The model under review builds one solid part; all positions refer to its coordinate system, in mm. Face numbers are marked on the shaded views. A direction names the side the tool comes from. Give positions to 0.01 mm unless a question says otherwise; leave off trailing zeros. Write each loop counter-clockwise with the first axis right and the second up, starting at its lowest first coordinate (ties: lowest second). Pieces come first, ordered by that corner, then holes. Notation, with made-up numbers: (2, 56.25) -> (28, 56.25) arc R22 ccw to (28, 70.25) -> close; hole circle Ø11 at (-8, 53). An arc over 180 degrees is marked (long way). Use CSV: the item, a comma, the result in double quotes.
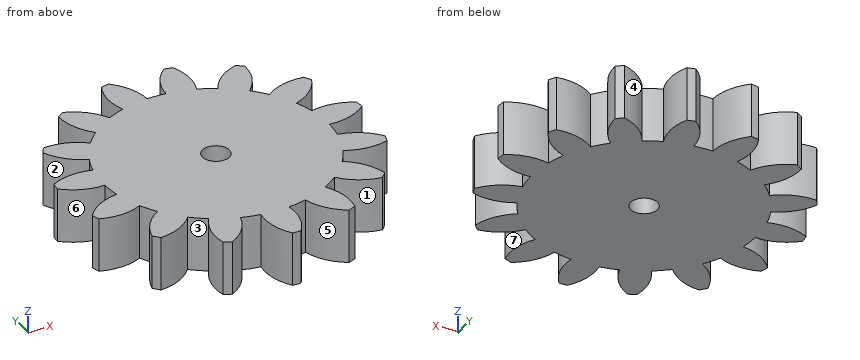
```python
from build123d import *

# Parameters (mm, degrees)
DODANIE_WYCI_GNI_CIE1_DEPTH = 12
OTW_R_6_0_6_1_D             = 6


with BuildPart() as part:
    # Szkic1 → Dodanie-wyciągnięcie1 (new body)
    with BuildSketch(Plane.XY):
        with BuildLine():
            ThreePointArc((-33.898094839, 2.630430818), (-29.769421597, 0.139315972), (-24.993476702, -0.525474417))
            ThreePointArc((-24.993476702, -0.525474417), (-24.862052862, -2.613107053), (-24.556561544, -4.68244446))
            ThreePointArc((-24.556561544, -4.68244446), (-29.089922891, -6.325682363), (-32.610442817, -9.620759807))
            ThreePointArc((-32.610442817, -9.620759807), (-32.335921554, -10.506577809), (-32.037343164, -11.384579176))
            ThreePointArc((-32.037343164, -11.384579176), (-27.252384788, -11.981043133), (-22.618947411, -10.645807579))
            ThreePointArc((-22.618947411, -10.645807579), (-21.649769069, -12.4995), (-20.529013513, -14.265679275))
            ThreePointArc((-20.529013513, -14.265679275), (-24.002080111, -17.610735974), (-25.87800636, -22.052863461))
            ThreePointArc((-25.87800636, -22.052863461), (-25.266924066, -22.750440616), (-24.637043805, -23.431092005))
            ThreePointArc((-24.637043805, -23.431092005), (-20.023163068, -22.029771036), (-16.333396627, -18.925383897))
            ThreePointArc((-16.333396627, -18.925383897), (-14.694043522, -20.224615842), (-12.951812545, -21.382248544))
            ThreePointArc((-12.951812545, -21.382248544), (-14.764059627, -25.850733346), (-14.671027508, -30.671826679))
            ThreePointArc((-14.671027508, -30.671826679), (-13.829045865, -31.06054556), (-12.976775752, -31.426156161))
            ThreePointArc((-12.976775752, -31.426156161), (-9.33175455, -28.269351393), (-7.223653181, -23.932589407))
            ThreePointArc((-7.223653181, -23.932589407), (-5.197584359, -24.452711871), (-3.135125524, -24.801632788))
            ThreePointArc((-3.135125524, -24.801632788), (-2.973199107, -29.620904076), (-0.927294719, -33.98735242))
            ThreePointArc((-0.927294719, -33.98735242), (0, -34), (0.927294719, -33.98735242))
            ThreePointArc((0.927294719, -33.98735242), (2.973199107, -29.620904076), (3.135125524, -24.801632788))
            ThreePointArc((3.135125524, -24.801632788), (5.197584359, -24.452711871), (7.223653181, -23.932589407))
            ThreePointArc((7.223653181, -23.932589407), (9.33175455, -28.269351393), (12.976775752, -31.426156161))
            ThreePointArc((12.976775752, -31.426156161), (13.829045865, -31.06054556), (14.671027508, -30.671826679))
            ThreePointArc((14.671027508, -30.671826679), (14.764059627, -25.850733346), (12.951812545, -21.382248544))
            ThreePointArc((12.951812545, -21.382248544), (14.694043522, -20.224615842), (16.333396627, -18.925383897))
            ThreePointArc((16.333396627, -18.925383897), (20.023163068, -22.029771036), (24.637043805, -23.431092005))
            ThreePointArc((24.637043805, -23.431092005), (25.266924066, -22.750440616), (25.87800636, -22.052863461))
            ThreePointArc((25.87800636, -22.052863461), (24.002080111, -17.610735974), (20.529013513, -14.265679275))
            ThreePointArc((20.529013513, -14.265679275), (21.649769069, -12.4995), (22.618947411, -10.645807579))
            ThreePointArc((22.618947411, -10.645807579), (27.252384788, -11.981043133), (32.037343164, -11.384579176))
            ThreePointArc((32.037343164, -11.384579176), (32.335921554, -10.506577809), (32.610442817, -9.620759807))
            ThreePointArc((32.610442817, -9.620759807), (29.089922891, -6.325682363), (24.556561544, -4.68244446))
            ThreePointArc((24.556561544, -4.68244446), (24.862052862, -2.613107053), (24.993476702, -0.525474417))
            ThreePointArc((24.993476702, -0.525474417), (29.769421597, 0.139315972), (33.898094839, 2.630430818))
            ThreePointArc((33.898094839, 2.630430818), (33.813744443, 3.553967751), (33.704237455, 4.47486062))
            ThreePointArc((33.704237455, 4.47486062), (29.14785373, 6.053139195), (24.338056995, 5.71042754))
            ThreePointArc((24.338056995, 5.71042754), (23.775461851, 7.725115842), (23.046406812, 9.685718046))
            ThreePointArc((23.046406812, 9.685718046), (27.139054966, 12.235586081), (29.897557962, 16.190615427))
            ThreePointArc((29.897557962, 16.190615427), (29.444863729, 17), (28.970263244, 17.796736993))
            ThreePointArc((28.970263244, 17.796736993), (24.165855859, 17.385317995), (19.911281288, 15.115914742))
            ThreePointArc((19.911281288, 15.115914742), (18.577877492, 16.727596028), (17.114403814, 18.222161866))
            ThreePointArc((17.114403814, 18.222161866), (19.81609918, 22.216212199), (20.727461703, 26.951295541))
            ThreePointArc((20.727461703, 26.951295541), (19.984698578, 27.506577809), (19.227067331, 28.041395862))
            ThreePointArc((19.227067331, 28.041395862), (15.00536197, 25.711417373), (12.041664157, 21.907722961))
            ThreePointArc((12.041664157, 21.907722961), (10.16800934, 22.837722896), (8.223164918, 23.607828357))
            ThreePointArc((8.223164918, 23.607828357), (9.066759823, 28.3554534), (7.973399012, 33.051851812))
            ThreePointArc((7.973399012, 33.051851812), (7.068997488, 33.257018425), (6.159336804, 33.437442638))
            ThreePointArc((6.159336804, 33.437442638), (3.250304677, 29.591779107), (2.089933898, 24.911486854))
            ThreePointArc((2.089933898, 24.911486854), (0, 24.999), (-2.089933898, 24.911486854))
            ThreePointArc((-2.089933898, 24.911486854), (-3.250304677, 29.591779107), (-6.159336804, 33.437442638))
            ThreePointArc((-6.159336804, 33.437442638), (-7.068997488, 33.257018425), (-7.973399012, 33.051851812))
            ThreePointArc((-7.973399012, 33.051851812), (-9.066759823, 28.3554534), (-8.223164918, 23.607828357))
            ThreePointArc((-8.223164918, 23.607828357), (-10.16800934, 22.837722896), (-12.041664157, 21.907722961))
            ThreePointArc((-12.041664157, 21.907722961), (-15.00536197, 25.711417373), (-19.227067331, 28.041395862))
            ThreePointArc((-19.227067331, 28.041395862), (-19.984698578, 27.506577809), (-20.727461703, 26.951295541))
            ThreePointArc((-20.727461703, 26.951295541), (-19.81609918, 22.216212199), (-17.114403814, 18.222161866))
            ThreePointArc((-17.114403814, 18.222161866), (-18.577877492, 16.727596028), (-19.911281288, 15.115914742))
            ThreePointArc((-19.911281288, 15.115914742), (-24.165855859, 17.385317995), (-28.970263244, 17.796736993))
            ThreePointArc((-28.970263244, 17.796736993), (-29.444863729, 17), (-29.897557962, 16.190615427))
            ThreePointArc((-29.897557962, 16.190615427), (-27.139054966, 12.235586081), (-23.046406812, 9.685718046))
            ThreePointArc((-23.046406812, 9.685718046), (-23.775461851, 7.725115842), (-24.338056995, 5.71042754))
            ThreePointArc((-24.338056995, 5.71042754), (-29.14785373, 6.053139195), (-33.704237455, 4.47486062))
            ThreePointArc((-33.704237455, 4.47486062), (-33.813744443, 3.553967751), (-33.898094839, 2.630430818))
        make_face()
    extrude(amount=DODANIE_WYCI_GNI_CIE1_DEPTH)

    # Otwór Ø6.0 (6)1 (through all)
    with Locations(Plane.XY.offset(12)):
        with Locations((0, 0)):
            Hole(OTW_R_6_0_6_1_D / 2)


solid = part.part
```
Q1. Consider section A-A (x = 0). Write out the cut boundary in (y, z), then the cut area to 3 significant figures.
Derived:
outline,"(-34, 0) -> (-3, 0) -> (-3, 12) -> (-34, 12) -> close; (3, 0) -> (25, 0) -> (25, 12) -> (3, 12) -> close"
area,"636 mm2"
Q2. Machinability: for the marked faces 1, 2 and 3, which of the approach directions +Z, -Z, +X, -X, +Y, -Y give a long, thin tool a straight path to every point of the face, cutting with its end or side? Answer none if there is none.
Derived:
face 1,"+Z, -Z, -Y"
face 2,"+Z, -Z, -X"
face 3,"+Z, -Z"
Q3. Consider section B-B (y = 1). Write out the cut boundary in (x, z), then the cut area to 3 significant figures.
Derived:
outline,"(-31.66, 0) -> (-2.83, 0) -> (-2.83, 12) -> (-31.66, 12) -> close; (2.83, 0) -> (31.66, 0) -> (31.66, 12) -> (2.83, 12) -> close"
area,"692 mm2"
Q4. Consider section C-C (y = -27). Write out the cut boundary in (x, z), then the cut area to 3 significant figures.
Derived:
outline,"(-14.92, 0) -> (-8.48, 0) -> (-8.48, 12) -> (-14.92, 12) -> close; (-3.3, 0) -> (3.3, 0) -> (3.3, 12) -> (-3.3, 12) -> close; (8.48, 0) -> (14.92, 0) -> (14.92, 12) -> (8.48, 12) -> close"
area,"234 mm2"
Q5. Insertion check: pin 1 (6 mm diameter, centred on x = 24.5, y = 7, fed in from -Z); pin 2 (3.5 mm diameter, centred on x = 0, y = 0, fed in from -Z). Each pin has a flat end and moves straight along its axis. Give the tip position at first contact, or say it passes through.
Derived:
pin 1,"stops at z = 0"
pin 2,"passes through"
Q6. To check wall thickness, follow probe 1 along Y at (x, z) = (0, 6); probe 2 along X at (y, z) = (-28, 1); probe 3 along X at (y, z) = (-21, 4.5). State the ranges of each line that lie inside material, in increasing order.
Derived:
probe 1,"y = -34 to -3, 3 to 25"
probe 2,"x = -14.96 to -9.13, -3.25 to 3.25, 9.13 to 14.96"
probe 3,"x = -25.62 to -18.44, -13.56 to 13.56, 18.44 to 25.62"
Q7. The part is to be moulded in two halves that separate along Y. For the marked faces 4, 5, 6 and 7, say which applies: pulls with the +Y half, pulls with the -Y half, needs draft (parallel to the pull), parting line crosses it, or undercut.
Derived:
face 4,"pulls with the +Y half"
face 5,"pulls with the -Y half"
face 6,"undercut"
face 7,"undercut"
Q8. Consider section D-D (y = -8.5). Write out the cut boundary in (x, z).
Derived:
outline,"(-31.71, 0) -> (31.71, 0) -> (31.71, 12) -> (-31.71, 12) -> close"
